The listing builds one solid part. Answer for the finished solid, in the listing's coordinates (mm). Coordinates: 2 decimals unless noted, no trailing zeros. Order: outer loops, then holes, each group sorted by start corner. A loop starts at its lowest first (then second) coordinate and runs counter-clockwise, first axis right, second up. Notation, with made-up numbers: (48, 12) -> (77, 12) arc R13 ccw to (77, 16) -> close; hole circle Ø3 at (41, 25). An arc over 180 degrees is marked (long way). Write each question's results on one line, items separated by ' | '. Start each with the question number.
(1) The part is cut by section B-B, the plane x = 20.32. Give the vertices of the cut face in (y, z), then the cut area to 3 significant figures.
(2) Straight lines are drawn through the part: L1, parallel to Y at x = 1.5, z = -42; L2, parallel to X at y = 29, z = -7; L3, parallel to X at y = 3.5, z = -33. For each, find the intervals that lie inside material, in ascending order.
(3) The part is cut by section A-A, the plane z = -7.62. Give the vertices of the cut face in (x, y).
(4) The part is cut by section D-D, the plane x = 2.5. Give the vertices of the cut face in (y, z), then the cut area to 3 significant figures.
(5) Given pin 1 (12 mm diameter, centred on y = 10.5, z = -49, fed in from +X); pin 2 (10 mm diameter, centred on y = 23.5, z = -28, fed in from +X); pin 3 (12 mm diameter, centred on x = 22.5, z = -58, fed in from +Y); pin 4 (6 mm diameter, centred on y = 25, z = -30, fed in from +X), each flat-ended and moving along its own axis, determine where each tip first touches the part or whether it passes through.
(6) Determine the mould class of faces 1 (the face through (21.751, 16.097, -3.077)), 2 (the face through (0, 16, -38)), 3 (the face through (3.174, 38.011, -72.243)), 4 (the face through (4, 44.45, -69)) for opening direction X: +X half, -X half, draft (parallel to the pull), parting line (faces both ways), or undercut.
```python
from build123d import *

# Parameters (mm, degrees)
BOSS_EXTRUDE1_DEPTH = 31.75
SKETCH2_R           = 4.7625
CUT_EXTRUDE2_DEPTH  = 89.44526556
SKETCH3_R           = 3.175
BOSS_EXTRUDE2_DEPTH = 12.7


with BuildPart() as part:
    # Sketch1 → Boss-Extrude1 (new body)
    with BuildSketch(Plane(origin=(0, 0, 0), x_dir=(1, 0, 0), z_dir=(0, 1, 0))):
        Polygon((0, 0), (0, 76.2), (6.35, 76.2), (31.75, 0), align=None)
    extrude(amount=BOSS_EXTRUDE1_DEPTH)

    # Sketch2 → Cut-Extrude2 (cut, through all)
    with BuildSketch(Plane(origin=(0, 31.75, 0), x_dir=(1, 0, 0), z_dir=(0, 1, 0))):
        with Locations(Location((20.32, 7.62, 0), (0, 0, 270))):
            Circle(SKETCH2_R)
    extrude(amount=-CUT_EXTRUDE2_DEPTH, mode=Mode.SUBTRACT)

    # Sketch3 → Boss-Extrude2 (add)
    with BuildSketch(Plane(origin=(0, 31.75, 0), x_dir=(1, 0, 0), z_dir=(0, 1, 0))):
        with Locations(Location((4.1275, 69.215, 0), (0, 0, 90))):
            Circle(SKETCH3_R)
    extrude(amount=BOSS_EXTRUDE2_DEPTH)


solid = part.part
```
Established:
1) outline: (0, -34.29) -> (31.75, -34.29) -> (31.75, -12.38) -> (0, -12.38) -> close; (0, -2.86) -> (31.75, -2.86) -> (31.75, 0) -> (0, 0) -> close | area: 786 mm^2
2) L1: y = 0 to 31.75 | L2: x = 0 to 15.6, 25.04 to 29.42 | L3: x = 0 to 20.75
3) outline: (0, 0) -> (15.56, 0) -> (15.56, 31.75) -> (0, 31.75) -> close; (25.08, 0) -> (29.21, 0) -> (29.21, 31.75) -> (25.08, 31.75) -> close
4) outline: (0, -76.2) -> (31.75, -76.2) -> (31.75, -71.94) -> (44.45, -71.94) -> (44.45, -66.49) -> (31.75, -66.49) -> (31.75, 0) -> (0, 0) -> close | area: 2,490 mm^2
5) pin 1: stops at x = 17.42 | pin 2: stops at x = 24.08 | pin 3: passes through | pin 4: stops at x = 22.75
6) face 1: undercut | face 2: -X half | face 3: parting line | face 4: draft
